```python
from build123d import *

# Parameters (mm, degrees)
SKETCH1_R           = 1
BOSS_EXTRUDE1_DEPTH = 2
SKETCH2_R           = 26.5
SKETCH2_R_2         = 25
BOSS_EXTRUDE2_DEPTH = 6
SKETCH3_R           = 17.5
CUT_EXTRUDE1_DEPTH  = 6


with BuildPart() as part:
    # Sketch1 → Boss-Extrude1 (new body)
    with BuildSketch(Plane.XY):
        with BuildLine():
            ThreePointArc((-19.463908256, 27.877522763), (-33.936185412, 2.082143047), (-22.725920861, -25.288980229))
            ThreePointArc((-22.725920861, -25.288980229), (-21.53176405, -32.517428202), (-14.410688779, -30.795000388))
            ThreePointArc((-14.410688779, -30.795000388), (15.164903933, -30.430670198), (33.263859745, -7.036734675))
            ThreePointArc((33.263859745, -7.036734675), (38.926800914, -2.388340554), (33.874597035, 2.917477625))
            ThreePointArc((33.874597035, 2.917477625), (18.771281479, 28.348527151), (-10.537938884, 32.325714904))
            ThreePointArc((-10.537938884, 32.325714904), (-17.395036864, 34.905768757), (-19.463908256, 27.877522763))
        make_face()
        with Locations((35.682900838, -2.189312175)):
            Circle(SKETCH1_R, mode=Mode.SUBTRACT)
        with Locations((-19.737450379, -29.807642519)):
            Circle(SKETCH1_R, mode=Mode.SUBTRACT)
        with Locations((-15.945450459, 31.996954694)):
            Circle(SKETCH1_R, mode=Mode.SUBTRACT)
    extrude(amount=BOSS_EXTRUDE1_DEPTH)

    # Sketch2 → Boss-Extrude2 (add)
    with BuildSketch(Plane.XY.offset(2)):
        Circle(SKETCH2_R)
        Circle(SKETCH2_R_2, mode=Mode.SUBTRACT)
    extrude(amount=BOSS_EXTRUDE2_DEPTH)

    # Sketch3 → Cut-Extrude1 (cut)
    with BuildSketch(Plane.XY.offset(2)):
        Circle(SKETCH3_R)
    extrude(amount=-CUT_EXTRUDE1_DEPTH, mode=Mode.SUBTRACT)


solid = part.part
```
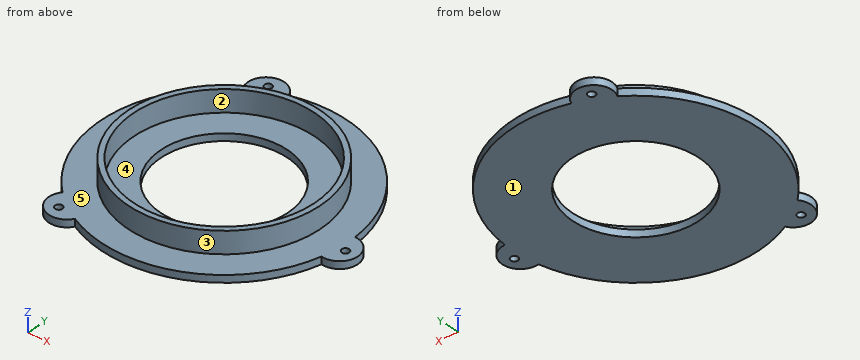
Here's how the part is built. I have some questions about the finished solid (model axes, mm). Face numbers are marked on the shaded views. A direction names the side the tool comes from. Coordinates: 2 decimals unless noted, no trailing zeros. Loops run counter-clockwise (first coordinate to the right, second up) from the corner with the lowest first, then second, coordinate; pieces in that order, holes last. Notation, with made-up numbers: M 1,0 L 25,0 A15 ccw 25,21 Z; hole C 41.25,-16.5 d1. An arc over 180 degrees is marked long. One line per item, written item: value.
1. Imagine slicing it at C-C (z = 3.5). List the corners of the cut face in (x, y) for me.
Geometry says:
outline: C 0,0 d53; hole C 0,0 d50
2. Imagine slicing it at B-B (y = 0). List the corners of the cut face in (x, z) for me.
Geometry says:
outline: M -34,0 L -17.5,0 L -17.5,2 L -25,2 L -25,8 L -26.5,8 L -26.5,2 L -34,2 Z; M 17.5,0 L 38.48,0 L 38.48,2 L 26.5,2 L 26.5,8 L 25,8 L 25,2 L 17.5,2 Z
3. Imagine slicing it at A-A (x = 0). List the corners of the cut face in (y, z) for me.
Geometry says:
outline: M -34,0 L -17.5,0 L -17.5,2 L -25,2 L -25,8 L -26.5,8 L -26.5,2 L -34,2 Z; M 17.5,0 L 34,0 L 34,2 L 26.5,2 L 26.5,8 L 25,8 L 25,2 L 17.5,2 Z
4. On a 3-axis mill with a long thin cutter (end or side, diameter ignored), from which of +Z, -Z, +X, -X, +Y, -Y can I reach the whole of each face in a straight line? I mean the marked faces 1 and 2. Say none if no direction works.
Geometry says:
face 1: -Z, +X, -X, +Y, -Y
face 2: +Z
5. Please list where these lines run through material, in increasing order: probe 1 along Y at (x, z) = (0, 0.9); probe 2 along Y at (x, z) = (0, 5.1); probe 3 along Z at (x, y) = (21, 8).
Geometry says:
probe 1: y = -34 to -17.5, 17.5 to 34
probe 2: y = -26.5 to -25, 25 to 26.5
probe 3: z = 0 to 2
6. Thinking about a two-plate mould opening in Y: for the marked faces 3, 4 and 5, which applies, +Y half, -Y half, draft (parallel to the pull), parting line (faces both ways), or undercut?
Geometry says:
face 3: parting line
face 4: undercut
face 5: draft
7. Imagine slicing it at D-D (y = -18.5). List the corners of the cut face in (x, z) for me, and give its area (3 significant figures).
Geometry says:
outline: M -28.53,0 L 28.53,0 L 28.53,2 L 18.97,2 L 18.97,8 L 16.82,8 L 16.82,2 L -16.82,2 L -16.82,8 L -18.97,8 L -18.97,2 L -28.53,2 Z
area: 140 mm2
8. Will these pins go through, and if not, where does the flat tip stop? pin 1 Ø1 at (y, z) = (11, 4) entering from -X; pin 2 Ø3 at (x, y) = (35.68, -2.19) entering from +Z; pin 3 Ø2 at (y, z) = (23.5, 6.5) entering from +X.
Geometry says:
pin 1: stops at x = -24.33
pin 2: stops at z = 2
pin 3: stops at x = 14
